Design review of the part built by this model. Coordinates are the model's own, in mm. Round coordinates to 2 decimals unless told otherwise and drop trailing zeros. Loops run counter-clockwise (first coordinate to the right, second up) from the corner with the lowest first, then second, coordinate; pieces in that order, holes last. Notation, with made-up numbers: M -25.5,-13.5 L 8.5,-13.5 A32 cw 8.5,14.5 Z; hole C 38,39.5 d1. An arc over 180 degrees is marked long. Use a Markdown table: item, result.
from build123d import *

# Parameters (mm, degrees)
BOSS_EXTRUDE1_DEPTH = 20
CHAMFER1_SIZE       = 2.5
SKETCH2_R           = 7.5
CUT_EXTRUDE1_DEPTH  = 85.852813742
CUT_EXTRUDE2_DEPTH  = 60
CUT_EXTRUDE3_DEPTH  = 85.852813742


with BuildPart() as part:
    # Sketch1 → Boss-Extrude1 (new body)
    with BuildSketch(Plane.XY):
        Polygon((0, 0), (0, 20), (20, 20), (20, 10), (80, 5), (80, 0), align=None)
    extrude(amount=BOSS_EXTRUDE1_DEPTH)

    # Chamfer1
    chamfer1_edges = [part.edges().sort_by_distance(p)[0] for p in [
        (50, 7.5, 20),
        (50, 7.5, 0),
    ]]
    chamfer(chamfer1_edges, length=CHAMFER1_SIZE)

    # Sketch2 → Cut-Extrude1 (cut, through all)
    with BuildSketch(Plane(origin=(0, 0, 0), x_dir=(-1, 0, 0), z_dir=(0, -1, 0))):
        with Locations(Location((-10, -10, 0), (0, 0, 90))):
            Circle(SKETCH2_R)
    extrude(amount=-CUT_EXTRUDE1_DEPTH, mode=Mode.SUBTRACT)

    # Sketch3 → Cut-Extrude2 (cut)
    with BuildSketch(Plane(origin=(80, 0, 0), x_dir=(0, 0, -1), z_dir=(1, 0, 0))):
        Polygon((-15, 2.199704526), (-16.27, 0), (-13.73, 0), align=None)
        Polygon((-6.27, 0), (-5, 2.199704526), (-3.73, 0), align=None)
    extrude(amount=-CUT_EXTRUDE2_DEPTH, mode=Mode.SUBTRACT)

    # Sketch4 → Cut-Extrude3 (cut, through all)
    with BuildSketch(Plane.XY):
        Polygon((75, 2.199704526), (73.73, 0), (76.27, 0), align=None)
        Polygon((65, 2.199704526), (63.73, 0), (66.27, 0), align=None)
        Polygon((50, 2.199704526), (48.73, 0), (51.27, 0), align=None)
        Polygon((35, 2.199704526), (33.73, 0), (36.27, 0), align=None)
    extrude(amount=CUT_EXTRUDE3_DEPTH, mode=Mode.SUBTRACT)


solid = part.part
1. Wall thickness on line 1 along X through (y, z) = (10.25, 10); line 2 along Z through (x, y) = (40, 2); line 3 along Z through (x, y) = (16.5, 7.5): over which ranges is each line inside the solid? List them lowest first. Write a range as from..to.
Check values:
| item | result |
|---|---|
| line 1 | x = 0..2.5, 17.5..20 |
| line 2 | z = 0..4.88, 5.12..14.88, 15.12..20 |
| line 3 | z = 0..6.26, 13.74..20 |
2. Take a section at A-A on z = 10. Give the boundary of the cut face in (x, y), and give its area (3 significant figures).
Check values:
| item | result |
|---|---|
| outline | M 0,0 L 2.5,0 L 2.5,20 L 0,20 Z; M 17.5,0 L 33.73,0 L 35,2.2 L 36.27,0 L 48.73,0 L 50,2.2 L 51.27,0 L 63.73,0 L 65,2.2 L 66.27,0 L 73.73,0 L 75,2.2 L 76.27,0 L 80,0 L 80,5 L 20,10 L 20,20 L 17.5,20 Z |
| area | 539 mm² |
3. Take a section at C-C on y = 8.5. Give the boundary of the cut face in (x, z), and give its area (3 significant figures).
Check values:
| item | result |
|---|---|
| outline | M 0,0 L 20,0 L 20,1.01 L 38,2.5 L 38,17.5 L 20,18.99 L 20,20 L 0,20 Z; hole C 10,10 d15 |
| area | 520 mm² |
4. Take a section at D-D on x = 68. Give the boundary of the cut face in (y, z), and give its area (3 significant figures).
Check values:
| item | result |
|---|---|
| outline | M 0,0 L 3.49,0 L 6,2.5 L 6,17.5 L 3.49,20 L 0,20 L 0,16.27 L 2.2,15 L 0,13.73 L 0,6.27 L 2.2,5 L 0,3.73 Z |
| area | 108 mm² |
5. Insertion check: pin 1 (2.5 mm diameter, centred on y = 1.5, z = 5, fed in from +X); pin 2 (6 mm diameter, centred on x = 58.5, z = 4.5, fed in from +Y); pin 3 (1.5 mm diameter, centred on x = 40, z = 10, fed in from +Y); pin 4 (3 mm diameter, centred on x = 45, z = 10.5, fed in from +Y). Each pin has a flat end and moves straight along its axis. Give the tip position at first contact, or say it passes through.
Check values:
| item | result |
|---|---|
| pin 1 | stops at x = 80 |
| pin 2 | stops at y = 7.04 |
| pin 3 | stops at y = 8.4 |
| pin 4 | stops at y = 8.04 |
6. The part is to be moulded in two halves that separate along X. For faces 1 (the face through (49.374, 1.115, 9.93)), 2 (the face through (20, 1, 5)), 3 (the face through (21, 0, 10)), say which applies: pulls with the +X half, pulls with the -X half, needs draft (parallel to the pull), parting line crosses it, or undercut.
Check values:
| item | result |
|---|---|
| face 1 | undercut |
| face 2 | pulls with the +X half |
| face 3 | needs draft |
7. Take a section at B-B on x = 10. Give the boundary of the cut face in (y, z).
Check values:
| item | result |
|---|---|
| outline | M 0,0 L 20,0 L 20,2.5 L 0,2.5 Z; M 0,17.5 L 20,17.5 L 20,20 L 0,20 Z |
